Here's how the part is built. I have some questions about the finished solid (model axes, mm). A direction names the side the tool comes from. Round coordinates to 2 decimals unless told otherwise and drop trailing zeros. Order: outer loops, then holes, each group sorted by start corner. A loop starts at its lowest first (then second) coordinate and runs counter-clockwise, first axis right, second up. Notation, with made-up numbers: (-0.75, -20.5) - (19.25, -20.5) arc R31 ccw to (19.25, 6.5) - close; hole circle Ø6 at (67.5, 72.5). An arc over 180 degrees is marked (long way). Answer as a JSON object with one key per item and string values.
```python
from build123d import *

# Parameters (mm, degrees)
SKETCH1_W                   = 20
SKETCH1_H                   = 10
BOSS_BODY_DEPTH             = 3.25
CUT_TOP_ANGLE_DEPTH         = 7.5
SKETCH3_W                   = 2
SKETCH3_H                   = 0.5
BOSS_BUTTON_DEPTH           = 1
BOSS_BUTTON_ROUND_TOP_DEPTH = 1
SKETCH5_R                   = 1.25
CUT_EXTRUDE2_DEPTH          = 7.5
SKETCH6_W                   = 3.2
SKETCH6_H                   = 5
BOSS_EXTRUDE4_DEPTH         = 0.5
EXTRUDE_THIN1_DEPTH         = 2


with BuildPart() as part:
    # Sketch1 → Boss-Body (new body, symmetric)
    with BuildSketch(Plane.XY):
        with Locations((0, 5)):
            Rectangle(SKETCH1_W, SKETCH1_H)
    extrude(amount=BOSS_BODY_DEPTH, both=True)

    # Sketch2 → Cut-Top Angle (cut, through all)
    with BuildSketch(Plane.XY.offset(3.25)):
        Polygon((1, 10), (-10, 9), (-10, 10), align=None)
    extrude(amount=-CUT_TOP_ANGLE_DEPTH, mode=Mode.SUBTRACT)

    # Sketch3 → Boss-Button (add, symmetric)
    with BuildSketch(Plane.XY):
        with Locations((3, 10.25)):
            Rectangle(SKETCH3_W, SKETCH3_H)
    extrude(amount=BOSS_BUTTON_DEPTH, both=True)

    # Sketch4 → Boss-Button Round Top (add, symmetric)
    with BuildSketch(Plane.XY):
        with BuildLine():
            Line((2, 10.5), (4, 10.5))
            ThreePointArc((4, 10.5), (3, 11.1), (2, 10.5))
        make_face()
    extrude(amount=BOSS_BUTTON_ROUND_TOP_DEPTH, both=True)

    # Sketch5 → Cut-Extrude2 (cut, through all)
    with BuildSketch(Plane.XY.offset(3.25)):
        with Locations((-4.75, 2)):
            Circle(SKETCH5_R)
        with Locations((4.75, 2)):
            Circle(SKETCH5_R)
    extrude(amount=-CUT_EXTRUDE2_DEPTH, mode=Mode.SUBTRACT)

    # Sketch6 → Boss-Extrude4 (add)
    with BuildSketch(Plane.XY):
        with Locations((-7.9, -2.5)):
            Rectangle(SKETCH6_W, SKETCH6_H)
        with Locations((7.9, -2.5)):
            Rectangle(SKETCH6_W, SKETCH6_H)
        with Locations((-0.6, -2.5)):
            Rectangle(SKETCH6_W, SKETCH6_H)
    extrude(amount=BOSS_EXTRUDE4_DEPTH)

    # Sketch7 → Extrude-Thin1 (add, symmetric)
    with BuildSketch(Plane.XY):
        Polygon((7.15, 10), (7.15, 10.630243429), (-9.563285177, 12.998516388), (-9.605374729, 12.701483612), (6.85, 10.369756571), (6.85, 10), align=None)
    extrude(amount=EXTRUDE_THIN1_DEPTH, both=True)


solid = part.part
```
1. Imagine slicing it at B-B (z = -2.25). List the corners of the cut face in (x, y) for me, plus the area to 3 significant figures.
Responses:
{"outline": "(-10, 0) - (10, 0) - (10, 10) - (1, 10) - (-10, 9) - close; hole circle Ø2.5 at (-4.75, 2); hole circle Ø2.5 at (4.75, 2)", "area": "185 mm2"}
2. Imagine slicing it at D-D (x = -7.5). List the corners of the cut face in (y, z) for me, plus the area to 3 significant figures.
Responses:
{"outline": "(-5, 0) - (0, 0) - (0, -3.25) - (9.23, -3.25) - (9.23, 3.25) - (0, 3.25) - (0, 0.5) - (-5, 0.5) - close; (12.4, -2) - (12.71, -2) - (12.71, 2) - (12.4, 2) - close", "area": "63.7 mm2"}
3. If I drill on L1, parallel to Y at x = -4.75, z = -0.5; L2, parallel to Y at x = -8.25, z = -1.5; L3, parallel to Y at x = 2.75, z = 2.5, over which ranges is the centre line in solid material (lowest first)? Write a range as [from, to].
Responses:
{"L1": "[0, 0.75], [3.25, 9.48], [12.01, 12.32]", "L2": "[0, 9.16], [12.51, 12.81]", "L3": "[0, 10]"}
4. For P1, Ø0.5, axis at x = 3, y = 10.5, coming from the +Z side; P2, Ø2, axis at x = 4.75, y = 2, coming from the -Z side; P3, Ø4, axis at x = -5, y = 9.5, coming from the -Z side; P4, Ø0.5, axis at y = 10.5, z = -0.5, coming from the +X side, each with a flat end and sliding along its axis, tell me the tip position at first contact or that it passes through.
Responses:
{"P1": "z = 1", "P2": "through", "P3": "z = -3.25", "P4": "x = 7.15"}
5. For faces 4 (the face through (-1, -2, 0)), 5 (the face through (3, 10.4, 1)), 6 (the face through (-1, -2, 0.5)), which set-ups out of +Z, -Z, +X, -X, +Y, -Y let a thin tool reach every point of the face, with its end or its side?
Responses:
{"face 4": "-Z, +X, -X, -Y", "face 5": "+Z, -X", "face 6": "+Z, +X, -X, -Y"}
6. Thinking about a two-plate mould opening in Y: for faces 1 (the face through (-4.423, 9.507, 0.046)), 2 (the face through (-1.1, 11.8, 0)), 3 (the face through (10, 5, 0)), which applies, pulls with the +Y half, pulls with the -Y half, needs draft (parallel to the pull), parting line crosses it, or undercut?
Responses:
{"face 1": "undercut", "face 2": "pulls with the +Y half", "face 3": "needs draft"}
7. Imagine slicing it at A-A (y = 2). List the corners of the cut face in (x, z) for me.
Responses:
{"outline": "(-10, -3.25) - (-6, -3.25) - (-6, 3.25) - (-10, 3.25) - close; (-3.5, -3.25) - (3.5, -3.25) - (3.5, 3.25) - (-3.5, 3.25) - close; (6, -3.25) - (10, -3.25) - (10, 3.25) - (6, 3.25) - close"}
8. Imagine slicing it at C-C (x = -4.25). List the corners of the cut face in (y, z) for me, plus the area to 3 significant figures.
Responses:
{"outline": "(0, -3.25) - (0.85, -3.25) - (0.85, 3.25) - (0, 3.25) - close; (3.15, -3.25) - (9.52, -3.25) - (9.52, 3.25) - (3.15, 3.25) - close; (11.94, -2) - (12.25, -2) - (12.25, 2) - (11.94, 2) - close", "area": "48.2 mm2"}
